Source: CAD feature listing. Evaluate the final solid. Frame: model axes, mm. A direction names the side the tool comes from. Give positions to 0.01 mm unless a question says otherwise; leave off trailing zeros. Write each loop counter-clockwise with the first axis right and the second up, starting at its lowest first coordinate (ties: lowest second). Pieces come first, ordered by that corner, then holes. Notation, with made-up numbers: (26, -36.75) -> (51, -36.75) arc R24 cw to (51, -11.75) -> close; hole circle Ø3 at (79.5, -17). An arc over 180 degrees is marked (long way). Answer as a JSON object with one key per item and string values. Group by question number.
Item 1: Access query for faces 1 (the face through (1, -2.146, 18)), 2 (the face through (2, 1.254, 18)), 3 (the face through (2, -0.646, 18)). Directions: +Z, -Z, +X, -X, +Y, -Y. A direction counts if a zero-diameter tool reaches every point of the face in a straight line with its end or side. Return the directions, or none.
Item 2: First-contact query: pin 1 Ø2 at (x, z) = (0.5, 19) entering from -Y; pin 2 Ø1.6 at (x, z) = (2.5, 17.5) entering from +Y; pin 3 Ø2 at (x, z) = (1, 19.5) entering from +Y. Flat tips, straight axial feed; report the tip coordinate or a pass-through.
Item 3: Section query A-A on x = -1.5. Return the cut outline in (y, z).
Item 4: Section query D-D on x = -2.5. Return the cut outline in (y, z), plus the area to 3 significant figures.
Item 5: Ray query, probe 1 along Z at (x, y) = (2.25, -1.5); probe 2 along X at (y, z) = (-1.5, 14.5); probe 3 along Y at (x, z) = (-1, 17). Return the intervals inside material, ascending. Write a range as from..to.
Item 6: Section query B-B on y = 2.25. Return the cut outline in (x, z).
Item 7: Section query C-C on z = 21.5. Return the cut outline in (x, y), plus the area to 3 significant figures.
Autodesk Inventor part; units mm, degrees
ref_plane "YZ Plane" through (0, 0, 0) normal (1, 0, 0) x (0, 1, 0)
ref_plane "XZ Plane" through (0, 0, 0) normal (0, 1, 0) x (-1, 0, 0)
ref_plane "XY Plane" through (0, 0, 0) normal (0, 0, 1) x (1, 0, 0)
sketch "Sketch1" plane through (0, 0, 0) normal (0, 0, 1) x (1, 0, 0)
  line L0 (-3.8602, 4.8039) -> (5.0398, 4.8039)
  line L1 (5.0398, 4.8039) -> (5.0398, -4.0961)
  line L2 (5.0398, -4.0961) -> (-3.8602, -4.0961)
  line L3 (-3.8602, -4.0961) -> (-3.8602, 4.8039)
  point P0 (0, 0)
  dimension "d0" = 8.9
  dimension "d1" = 8.9
extrude "Extrusion1" add sketch "Sketch1" along normal blind 13
sketch "Sketch2" plane through (0, 0, 13) normal (0, 0, 1) x (1, 0, 0)
  line L0 (-0.3102, 2.7539) -> (1.5898, 2.7539)
  line L1 (1.5898, -2.1461) -> (-0.3102, -2.1461)
  line L2 (3.0898, 1.2539) -> (3.0898, -0.6461)
  line L3 (-1.8102, -0.6461) -> (-1.8102, 1.2539)
  line L4 (-3.8602, 4.8039) -> (5.0398, 4.8039)
  line L5 (-3.8602, -4.0961) -> (-3.8602, 4.8039)
  line L6 (5.0398, 4.8039) -> (5.0398, -4.0961)
  line L7 (-3.8602, -4.0961) -> (5.0398, -4.0961)
  line L8 (-1.8102, 1.2539) -> (-0.3102, 1.2539)
  line L9 (1.5898, 1.2539) -> (3.0898, 1.2539)
  line L10 (-0.3102, -2.1461) -> (-0.3102, -0.6461)
  line L11 (-0.3102, 1.2539) -> (-0.3102, 2.7539)
  line L12 (3.0898, -0.6461) -> (1.5898, -0.6461)
  line L13 (-0.3102, -0.6461) -> (-1.8102, -0.6461)
  line L14 (1.5898, 2.7539) -> (1.5898, 1.2539)
  line L15 (1.5898, -0.6461) -> (1.5898, -2.1461)
  point P0 (0, 0)
  dimension "d4" = 1.9
  dimension "d5" = 1.9
  dimension "d6" = 4.9
  dimension "d7" = 4.9
extrude "Extrusion2" add sketch "Sketch2" along normal blind 10 contours L0 L14 L9 L2 L12 L15 L1 L10 L13 L3 L8 L11
properties part number "ClutchAdapter"
Worked answers:
{
 "1": {"face 1": "+Z, +X, -X, -Y", "face 2": "+Z, +X, +Y", "face 3": "+Z, +X, -Y"},
 "2": {"pin 1": "y = -2.15", "pin 2": "y = 1.25", "pin 3": "y = 2.75"},
 "3": {"outline": "(-4.1, 0) -> (4.8, 0) -> (4.8, 13) -> (1.25, 13) -> (1.25, 23) -> (-0.65, 23) -> (-0.65, 13) -> (-4.1, 13) -> close"},
 "4": {"outline": "(-4.1, 0) -> (4.8, 0) -> (4.8, 13) -> (-4.1, 13) -> close", "area": "116 mm^2"},
 "5": {"probe 1": "0..13", "probe 2": "-0.31..1.59", "probe 3": "-0.65..1.25"},
 "6": {"outline": "(-3.86, 0) -> (5.04, 0) -> (5.04, 13) -> (1.59, 13) -> (1.59, 23) -> (-0.31, 23) -> (-0.31, 13) -> (-3.86, 13) -> close"},
 "7": {"outline": "(-1.81, -0.65) -> (-0.31, -0.65) -> (-0.31, -2.15) -> (1.59, -2.15) -> (1.59, -0.65) -> (3.09, -0.65) -> (3.09, 1.25) -> (1.59, 1.25) -> (1.59, 2.75) -> (-0.31, 2.75) -> (-0.31, 1.25) -> (-1.81, 1.25) -> close", "area": "15.0 mm^2"}
}
